Source: CAD feature listing. Evaluate the final solid. Frame: model axes, mm. Round coordinates to 2 decimals unless told otherwise and drop trailing zeros. Write each loop counter-clockwise with the first axis right and the second up, starting at its lowest first coordinate (ties: lowest second). Pieces come first, ordered by that corner, then holes. Notation, with made-up numbers: M -25.75,-28.75 L -13.75,-28.75 A18 cw -13.75,-9.75 Z; hole C 14.5,41 d11. An arc over 180 degrees is marked long. Use a Markdown table: item, result.
```python
from build123d import *

# Parameters (mm, degrees)
ESQUISSE1_R        = 6
ESQUISSE1_R_2      = 4
BOSS_EXTRU_1_DEPTH = 10
CHANFREIN1_SIZE    = 0.2


with BuildPart() as part:
    # Esquisse1 → Boss.-Extru.1 (new body)
    with BuildSketch(Plane.XY):
        Circle(ESQUISSE1_R)
        Circle(ESQUISSE1_R_2, mode=Mode.SUBTRACT)
    extrude(amount=BOSS_EXTRU_1_DEPTH)

    # Chanfrein1
    chanfrein1_edges = [part.edges().sort_by_distance(p)[0] for p in [
        (-6, 0, 0),
        (-6, 0, 10),
        (-4, 0, 0),
        (-4, 0, 10),
    ]]
    chamfer(chanfrein1_edges, length=CHANFREIN1_SIZE)


solid = part.part
```
Q1. Line query: L1, parallel to Y at x = 0, z = 3.75; L2, parallel to Y at x = -2.75, z = 3.5; L3, parallel to X at y = 0.75, z = 2. Output: solid intervals per line, ascending.
Results are:
| item | result |
|---|---|
| L1 | -6 to -4, 4 to 6 |
| L2 | -5.33 to -2.9, 2.9 to 5.33 |
| L3 | -5.95 to -3.93, 3.93 to 5.95 |
Q2. Section A-A on x = 0. Return loops of the section in (y, z), plus the area to 3 significant figures.
Results are:
| item | result |
|---|---|
| outline | M -6,0.2 L -5.8,0 L -4.2,0 L -4,0.2 L -4,9.8 L -4.2,10 L -5.8,10 L -6,9.8 Z; M 4,0.2 L 4.2,0 L 5.8,0 L 6,0.2 L 6,9.8 L 5.8,10 L 4.2,10 L 4,9.8 Z |
| area | 39.8 mm^2 |
Q3. Section C-C on z = 8. Return loops of the section in (x, y).
Results are:
| item | result |
|---|---|
| outline | C 0,0 d12; hole C 0,0 d8 |
Q4. Mould query, pull axis X, two halves, no side actions, for faces 1 (the cylindrical face through (-6, 0, 5)), 2 (the flat face through (4, 2, 10)), 3 (the cylindrical face through (-0.867, -3.905, 4.933)). Classes: +X half, -X half, draft (parallel to the pull), parting line (faces both ways), or undercut.
Results are:
| item | result |
|---|---|
| face 1 | parting line |
| face 2 | draft |
| face 3 | undercut |
Q5. First-contact query: pin 1 Ø4 at (x, z) = (-1.5, 7) entering from +Y; pin 2 Ø6 at (x, z) = (-4.5, 6.5) entering from +Y. Flat tips, straight axial feed; report the tip coordinate or a pass-through.
Results are:
| item | result |
|---|---|
| pin 1 | y = 6 |
| pin 2 | y = 5.81 |
